Answer from the drawing. Dimensions are ordinates in mm from the lowest x, y and z of the part. Round coordinates to 2 decimals unless told otherwise and drop trailing zeros. Order: outer loops, then holes, each group sorted by start corner. A loop starts at its lowest first (then second) coordinate and runs counter-clockwise, first axis right, second up. Notation, with made-up numbers: M -33,21 L 22,21 A24 cw 22,55 Z; hole C 37.25,-29 d3. An arc over 180 degrees is marked long. Use one line per item in the form item = value. Start each with the question number.
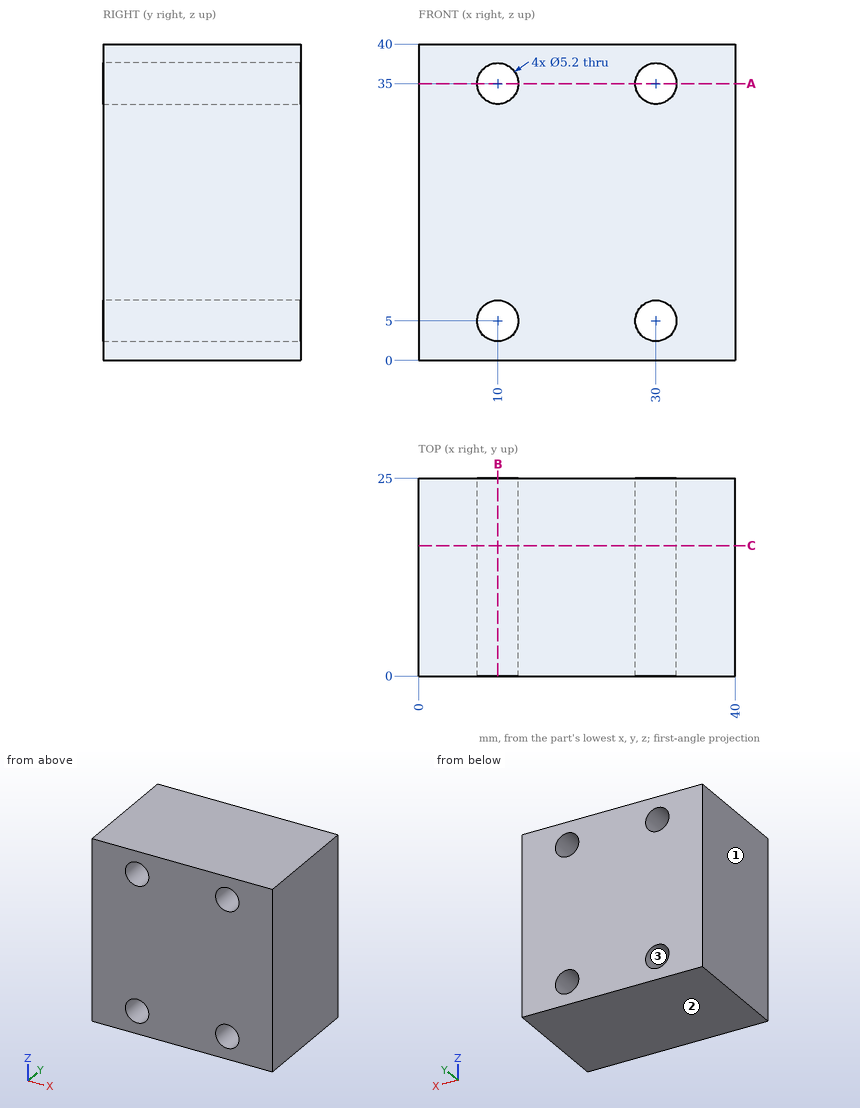
Item 1: Section C-C (y = 16.5) is taken. Write down the section's boundary in (x, z), and give its area (3 significant figures).
Item 2: Find the intervals of material crossed by L1, parallel to X at y = 13.75, z = 35; L2, parallel to Z at x = 12, y = 1.75; L3, parallel to X at y = 14, z = 3, in increasing order. Write a range as [from, to].
Item 3: Given P1, Ø2, axis at x = 33.5, z = 31, coming from the -Y side; P2, Ø4, axis at x = 30, z = 5, coming from the +Y side, each flat-ended and moving along its own axis, determine where each tip first touches the part or whether it passes through.
Item 4: Section B-B (x = 10) is taken. Write down the section's boundary in (y, z), and give its area (3 significant figures).
Item 5: For a pull along X with two mould halves and no side action, classify the marked faces 1, 2 and 3 as pulls with the +X half, pulls with the -X half, needs draft (parallel to the pull), parting line crosses it, or undercut.
Item 6: Section A-A (z = 35) is taken. Write down the section's boundary in (x, y).
The answers:
q1.outline = M 0,0 L 40,0 L 40,40 L 0,40 Z; hole C 10,5 d5.2; hole C 10,35 d5.2; hole C 30,5 d5.2; hole C 30,35 d5.2
q1.area = 1,520 mm²
q2.L1 = [0, 7.4], [12.6, 27.4], [32.6, 40]
q2.L2 = [0, 3.34], [6.66, 33.34], [36.66, 40]
q2.L3 = [0, 8.34], [11.66, 28.34], [31.66, 40]
q3.P1 = 0
q3.P2 = through
q4.outline = M 0,0 L 25,0 L 25,2.4 L 0,2.4 Z; M 0,7.6 L 25,7.6 L 25,32.4 L 0,32.4 Z; M 0,37.6 L 25,37.6 L 25,40 L 0,40 Z
q4.area = 740 mm²
q5.face_1 = pulls with the -X half
q5.face_2 = needs draft
q5.face_3 = undercut
q6.outline = M 0,0 L 7.4,0 L 7.4,25 L 0,25 Z; M 12.6,0 L 27.4,0 L 27.4,25 L 12.6,25 Z; M 32.6,0 L 40,0 L 40,25 L 32.6,25 Z
